from build123d import *

# Parameters (mm, degrees)
IZIM1_R                     = 60
IZIM1_R_2                   = 1.75
Y_KSEKLIK_EKSTR_ZYON1_DEPTH = 2
IZIM2_R                     = 1.75
KES_EKSTR_ZYON1_DEPTH       = 10
IZIM3_R                     = 25
KES_EKSTR_ZYON2_DEPTH       = 10


with BuildPart() as part:
    # Çizim1 → Yükseklik-Ekstrüzyon1 (new body)
    with BuildSketch(Plane(origin=(0, 0, 0), x_dir=(1, 0, 0), z_dir=(0, 1, 0))):
        with Locations(Location((0, 0, 0), (0, 0, 270))):
            Circle(IZIM1_R)
        with Locations(Location((-51.576054603, 18.772148676, 0), (0, 0, 270))):
            Circle(IZIM1_R_2, mode=Mode.SUBTRACT)
        with Locations(Location((-18.712348032, 51.411753683, 0), (0, 0, 270))):
            Circle(IZIM1_R_2, mode=Mode.SUBTRACT)
        with Locations(Location((18.772148676, 51.576054603, 0), (0, 0, 270))):
            Circle(IZIM1_R_2, mode=Mode.SUBTRACT)
        with Locations(Location((51.411753683, 18.712348032, 0), (0, 0, 270))):
            Circle(IZIM1_R_2, mode=Mode.SUBTRACT)
        with Locations(Location((51.576054603, -18.772148676, 0), (0, 0, 270))):
            Circle(IZIM1_R_2, mode=Mode.SUBTRACT)
        with Locations(Location((18.712348032, -51.411753683, 0), (0, 0, 270))):
            Circle(IZIM1_R_2, mode=Mode.SUBTRACT)
        with Locations(Location((-18.772148676, -51.576054603, 0), (0, 0, 270))):
            Circle(IZIM1_R_2, mode=Mode.SUBTRACT)
        with Locations(Location((-51.411753683, -18.712348032, 0), (0, 0, 270))):
            Circle(IZIM1_R_2, mode=Mode.SUBTRACT)
    extrude(amount=Y_KSEKLIK_EKSTR_ZYON1_DEPTH)

    # Çizim2 → Kes-Ekstrüzyon1 (cut)
    with BuildSketch(Plane(origin=(0, 2, 0), x_dir=(1, 0, 0), z_dir=(0, 1, 0))):
        with Locations(Location((0, 35, 0), (0, 0, 270))):
            Circle(IZIM2_R)
        with Locations(Location((35, 0, 0), (0, 0, 270))):
            Circle(IZIM2_R)
        with Locations(Location((0, -35, 0), (0, 0, 270))):
            Circle(IZIM2_R)
        with Locations(Location((-35, 0, 0), (0, 0, 270))):
            Circle(IZIM2_R)
    extrude(amount=-KES_EKSTR_ZYON1_DEPTH, mode=Mode.SUBTRACT)

    # Çizim3 → Kes-Ekstrüzyon2 (cut)
    with BuildSketch(Plane(origin=(0, 2, 0), x_dir=(1, 0, 0), z_dir=(0, 1, 0))):
        with Locations(Location((0, 0, 0), (0, 0, 270))):
            Circle(IZIM3_R)
    extrude(amount=-KES_EKSTR_ZYON2_DEPTH, mode=Mode.SUBTRACT)


solid = part.part
Could you check a few things on this model? Use its own coordinates, in mm. Coordinates: 2 decimals unless noted, no trailing zeros. Order: outer loops, then holes, each group sorted by start corner. A loop starts at its lowest first (then second) coordinate and runs counter-clockwise, first axis right, second up.
Q1. Suppose I cut it at D-D on x = 35. Please give me the cut outline in (y, z), and give its area (3 significant figures).
Q2. Will these pins go through, and if not, where does the flat tip stop? pin 1 (3 mm diameter, centred on x = -35, z = 0, fed in from -Y); pin 2 (1 mm diameter, centred on x = 40.5, y = 1, fed in from -Z).
Q3. Please list where these lines run through material, in increasing order: L1, parallel to X at y = 1.2, z = 0; L2, parallel to Z at x = -18.5, y = 1.25; L3, parallel to Z at x = 7, y = 0.4.
Q4. Suppose I cut it at B-B on z = 0. Please give me the cut outline in (x, y).
Q5. Suppose I cut it at C-C on z = 35. Please give me the cut outline in (x, y), and give its area (3 significant figures).
Q6. Thinking about a two-plate mould opening in X: for faces 1 (the cylindrical face through (2.64, 0.99, -59.94)), 2 (the cylindrical face through (53.31, 0.99, 18.54)), 3 (the flat face through (1, 2, 26)), which applies, released by +X, released by -X, zero draft, split by the parting line, or undercut?
Q7. Suppose I cut it at A-A on x = 0. Please give me the cut outline in (y, z).
Answer:
1. outline: (0, -48.73) - (2, -48.73) - (2, -1.75) - (0, -1.75) - close; (0, 1.75) - (2, 1.75) - (2, 48.73) - (0, 48.73) - close
1. area: 188 mm2
2. pin 1: passes through
2. pin 2: stops at z = -44.72
3. L1: x = -60 to -36.75, -33.25 to -25, 25 to 33.25, 36.75 to 60
3. L2: z = -57.08 to -53.15, -49.67 to -16.82, 16.82 to 49.85, 53.3 to 57.08
3. L3: z = -59.59 to -24, 24 to 59.59
4. outline: (-60, 0) - (-36.75, 0) - (-36.75, 2) - (-60, 2) - close; (-33.25, 0) - (-25, 0) - (-25, 2) - (-33.25, 2) - close; (25, 0) - (33.25, 0) - (33.25, 2) - (25, 2) - close; (36.75, 0) - (60, 0) - (60, 2) - (36.75, 2) - close
5. outline: (-48.73, 0) - (-1.75, 0) - (-1.75, 2) - (-48.73, 2) - close; (1.75, 0) - (48.73, 0) - (48.73, 2) - (1.75, 2) - close
5. area: 188 mm2
6. face 1: split by the parting line
6. face 2: undercut
6. face 3: zero draft
7. outline: (0, -60) - (2, -60) - (2, -36.75) - (0, -36.75) - close; (0, -33.25) - (2, -33.25) - (2, -25) - (0, -25) - close; (0, 25) - (2, 25) - (2, 33.25) - (0, 33.25) - close; (0, 36.75) - (2, 36.75) - (2, 60) - (0, 60) - close
